Read the model definition and answer for the solid it produces. Units are mm, in the model's axes. A direction names the side the tool comes from. Give positions to 0.01 mm unless a question says otherwise; leave off trailing zeros. Order: outer loops, then holes, each group sorted by start corner. A loop starts at its lowest first (then second) coordinate and runs counter-clockwise, first axis right, second up. Notation, with made-up numbers: M 54.5,16.5 L 80.5,16.5 A13 cw 80.5,28.5 Z; hole C 87,30.25 d10. An arc over 180 degrees is marked long. One line per item, written item: value. Start each with the question number.
from build123d import *

# Parameters (mm, degrees)
SKETCH_1_R          = 1
EXTRUDE_1_DEPTH     = 1.6
SKETCH_3_R          = 1.5
CUT_EXTRUDE_1_DEPTH = 1.6
CUT_EXTRUDE_2_DEPTH = 1.6
EXTRUDE_2_DEPTH     = 1.6
SKETCH_8_W          = 1.78
SKETCH_8_H          = 8.1
CUT_EXTRUDE_3_DEPTH = 0.1
CUT_EXTRUDE_START   = 1.6
SKETCH_9_W          = 1.78
SKETCH_9_H          = 8.1
CUT_EXTRUDE_4_DEPTH = 0.1
EXTRUDE_START       = 1.6
EXTRUDE_3_DEPTH     = 1.6
SKETCH_12_W         = 1.78
SKETCH_12_H         = 8.1
CUT_EXTRUDE_5_DEPTH = 0.1
SKETCH_13_W         = 1.78
SKETCH_13_H         = 8.1
CUT_EXTRUDE_6_DEPTH = 0.1


with BuildPart() as part:
    # 草图1 → 凸台-拉伸1 (new body)
    with BuildSketch(Plane.XY):
        with BuildLine():
            Line((-9.15, 16), (9.15, 16))
            ThreePointArc((9.15, 16), (10.458147545, 15.458147545), (11, 14.15))
            Line((11, 14.15), (11, -20))
            Line((11, -20), (-11, -20))
            Line((-11, -20), (-11, 14.15))
            ThreePointArc((-11, 14.15), (-10.458147545, 15.458147545), (-9.15, 16))
        make_face()
        with Locations((-9.15, 14.15)):
            Circle(SKETCH_1_R, mode=Mode.SUBTRACT)
        with Locations((9.15, 14.15)):
            Circle(SKETCH_1_R, mode=Mode.SUBTRACT)
    extrude(amount=EXTRUDE_1_DEPTH)

    # 草图3 → 切除-拉伸1 (cut)
    with BuildSketch(Plane.XY):
        with Locations((-7.5, -17.5)):
            Circle(SKETCH_3_R)
        with Locations((7.5, -17.5)):
            Circle(SKETCH_3_R)
    extrude(amount=CUT_EXTRUDE_1_DEPTH, mode=Mode.SUBTRACT)

    # 草图5 → 切除-拉伸2 (cut)
    with BuildSketch(Plane.XY):
        with BuildLine():
            Line((11, -20), (11, -18.15))
            ThreePointArc((11, -18.15), (10.458147545, -19.458147545), (9.15, -20))
            Line((9.15, -20), (11, -20))
        make_face()
        with BuildLine():
            Line((-11, -20), (-9.15, -20))
            ThreePointArc((-9.15, -20), (-10.458147545, -19.458147545), (-11, -18.15))
            Line((-11, -18.15), (-11, -20))
        make_face()
    extrude(amount=CUT_EXTRUDE_2_DEPTH, mode=Mode.SUBTRACT)

    # 草图7 → 凸台-拉伸2 (add)
    with BuildSketch(Plane.XY):
        with BuildLine():
            Line((-4.915, 26.92), (4.915, 26.92))
            ThreePointArc((4.915, 26.92), (5.975660172, 26.480660172), (6.415, 25.42))
            Line((6.415, 25.42), (6.415, 16))
            Line((6.415, 16), (-6.415, 16))
            Line((-6.415, 16), (-6.415, 25.42))
            ThreePointArc((-6.415, 25.42), (-5.975660172, 26.480660172), (-4.915, 26.92))
        make_face()
        with BuildLine():
            Line((-6.415, -20), (6.415, -20))
            Line((6.415, -20), (6.415, -29.42))
            ThreePointArc((6.415, -29.42), (5.975660172, -30.480660172), (4.915, -30.92))
            Line((4.915, -30.92), (-4.915, -30.92))
            ThreePointArc((-4.915, -30.92), (-5.975660172, -30.480660172), (-6.415, -29.42))
            Line((-6.415, -29.42), (-6.415, -20))
        make_face()
    extrude(amount=EXTRUDE_2_DEPTH)

    # 草图8 → 切除-拉伸3 (cut)
    with BuildSketch(Plane.XY):
        with Locations((-1.27, 22.37)):
            Rectangle(SKETCH_8_W, SKETCH_8_H)
        with Locations((-3.81, 22.37)):
            Rectangle(SKETCH_8_W, SKETCH_8_H)
        with Locations((3.81, 22.37)):
            Rectangle(SKETCH_8_W, SKETCH_8_H)
        with Locations((1.27, 22.37)):
            Rectangle(SKETCH_8_W, SKETCH_8_H)
        with Locations((1.27, -26.37)):
            Rectangle(SKETCH_8_W, SKETCH_8_H)
        with Locations((3.81, -26.37)):
            Rectangle(SKETCH_8_W, SKETCH_8_H)
        with Locations((-3.81, -26.37)):
            Rectangle(SKETCH_8_W, SKETCH_8_H)
        with Locations((-1.27, -26.37)):
            Rectangle(SKETCH_8_W, SKETCH_8_H)
    extrude(amount=CUT_EXTRUDE_3_DEPTH, mode=Mode.SUBTRACT)

    # 草图9 → 切除-拉伸4 (cut)
    with BuildSketch(Plane.XY.offset(CUT_EXTRUDE_START)):
        with Locations((-1.27, 22.37)):
            Rectangle(SKETCH_9_W, SKETCH_9_H)
        with Locations((1.27, 22.37)):
            Rectangle(SKETCH_9_W, SKETCH_9_H)
        with Locations((3.81, 22.37)):
            Rectangle(SKETCH_9_W, SKETCH_9_H)
        with Locations((-3.81, 22.37)):
            Rectangle(SKETCH_9_W, SKETCH_9_H)
        with Locations((-1.27, -26.37)):
            Rectangle(SKETCH_9_W, SKETCH_9_H)
        with Locations((-3.81, -26.37)):
            Rectangle(SKETCH_9_W, SKETCH_9_H)
        with Locations((3.81, -26.37)):
            Rectangle(SKETCH_9_W, SKETCH_9_H)
        with Locations((1.27, -26.37)):
            Rectangle(SKETCH_9_W, SKETCH_9_H)
    extrude(amount=-CUT_EXTRUDE_4_DEPTH, mode=Mode.SUBTRACT)

    # 草图11 → 凸台-拉伸3 (add)
    with BuildSketch(Plane.XY.offset(EXTRUDE_START)):
        with BuildLine():
            Line((-7.62, -20), (7.62, -20))
            Line((7.62, -20), (7.62, -29.42))
            ThreePointArc((7.62, -29.42), (7.180660172, -30.480660172), (6.12, -30.92))
            Line((6.12, -30.92), (-6.12, -30.92))
            ThreePointArc((-6.12, -30.92), (-7.180660172, -30.480660172), (-7.62, -29.42))
            Line((-7.62, -29.42), (-7.62, -20))
        make_face()
    extrude(amount=-EXTRUDE_3_DEPTH)

    # 草图12 → 切除-拉伸5 (cut)
    with BuildSketch(Plane.XY):
        with Locations((0, -26.37)):
            Rectangle(SKETCH_12_W, SKETCH_12_H)
        with Locations((2.54, -26.37)):
            Rectangle(SKETCH_12_W, SKETCH_12_H)
        with Locations((5.08, -26.37)):
            Rectangle(SKETCH_12_W, SKETCH_12_H)
        with Locations((-2.54, -26.37)):
            Rectangle(SKETCH_12_W, SKETCH_12_H)
        with Locations((-5.08, -26.37)):
            Rectangle(SKETCH_12_W, SKETCH_12_H)
    extrude(amount=CUT_EXTRUDE_5_DEPTH, mode=Mode.SUBTRACT)

    # 草图13 → 切除-拉伸6 (cut)
    with BuildSketch(Plane.XY.offset(CUT_EXTRUDE_START)):
        with Locations((2.54, -26.37)):
            Rectangle(SKETCH_13_W, SKETCH_13_H)
        with Locations((0, -26.37)):
            Rectangle(SKETCH_13_W, SKETCH_13_H)
        with Locations((-5.08, -26.37)):
            Rectangle(SKETCH_13_W, SKETCH_13_H)
        with Locations((-2.54, -26.37)):
            Rectangle(SKETCH_13_W, SKETCH_13_H)
        with Locations((5.08, -26.37)):
            Rectangle(SKETCH_13_W, SKETCH_13_H)
    extrude(amount=-CUT_EXTRUDE_6_DEPTH, mode=Mode.SUBTRACT)


solid = part.part
Q1. A tool of negligible diameter and unlimited length cuts with its end or side. For faces 1 (the flat face through (-8, -20, 1)), 2 (the flat face through (-3, -26, 0.1)), 3 (the flat face through (-8, 16, 1)), 4 (the flat face through (1, 22, 1.5)), from which of +Z, -Z, +X, -X, +Y, -Y can it reach the whole face along a straight path? Write none if from no direction.
Q2. Each of these flat-tipped pins is pushed along its axis until it touches: pin 1 (1.8 mm diameter, centred on x = -9.15, y = 14.15, fed in from -Z); pin 2 (0.5 mm diameter, centred on x = -3, y = -26, fed in from +Z). Where does it stop, or does it pass through?
Q3. Determine the mould class of faces 5 (the cylindrical face through (8.413, 14.826, 0.789)), 6 (the flat face through (8, -20, 1)), 7 (the cylindrical face through (5.964, 26.492, 0.789)) for opening direction Y: released by +Y, released by -Y, zero draft, split by the parting line, or undercut.
Q4. Find section A-A, the plane z = 0.8. Give the vertices of the cut face in (x, y) (3 decimals), then the cut area to 3 significant figures.
Q5. Consider probe 1 along Y at (x, z) = (-9.15, 0.95); probe 2 along X at (y, z) = (19.5, 0.55) (3 decimals); probe 3 along Z at (x, y) = (1.75, -26.5). Determine where each line is inside the solid, lowest interval first.
Q6. Find section B-B, the plane y = -17.5. Give the vertices of the cut face in (x, z), then the cut area to 3 significant figures.
Evaluation:
1. face 1: +Z, -Z, -X, -Y
1. face 2: -Z
1. face 3: +Z, -Z, -X, +Y
1. face 4: +Z
2. pin 1: through
2. pin 2: z = 1.5
3. face 5: undercut
3. face 6: released by -Y
3. face 7: released by +Y
4. outline: M -11,-18.15 A1.85 ccw -9.15,-20 L -7.62,-20 L -7.62,-29.42 A1.5 ccw -6.12,-30.92 L 6.12,-30.92 A1.5 ccw 7.62,-29.42 L 7.62,-20 L 9.15,-20 A1.85 ccw 11,-18.15 L 11,14.15 A1.85 ccw 9.15,16 L 6.415,16 L 6.415,25.42 A1.5 ccw 4.915,26.92 L -4.915,26.92 A1.5 ccw -6.415,25.42 L -6.415,16 L -9.15,16 A1.85 ccw -11,14.15 Z; hole C -9.15,14.15 d2; hole C -7.5,-17.5 d3; hole C 7.5,-17.5 d3; hole C 9.15,14.15 d2
4. area: 1,070 mm2
5. probe 1: -20 to 13.15, 15.15 to 16
5. probe 2: -6.415 to 6.415
5. probe 3: 0.1 to 1.5
6. outline: M -11,0 L -9,0 L -9,1.6 L -11,1.6 Z; M -6,0 L 6,0 L 6,1.6 L -6,1.6 Z; M 9,0 L 11,0 L 11,1.6 L 9,1.6 Z
6. area: 25.6 mm2
